Model file for the job. Use its own axes, mm. Face numbers are marked on the shaded views. A direction names the side the tool comes from. Give positions to 0.01 mm unless a question says otherwise; leave off trailing zeros. Write each loop counter-clockwise with the first axis right and the second up, starting at its lowest first coordinate (ties: lowest second). Pieces come first, ordered by that corner, then holes.
Autodesk Inventor part; units mm, degrees
ref_plane "YZ Plane" through (0, 0, 0) normal (1, 0, 0) x (0, 1, 0)
ref_plane "XZ Plane" through (0, 0, 0) normal (0, 1, 0) x (-1, 0, 0)
ref_plane "XY Plane" through (0, 0, 0) normal (0, 0, 1) x (1, 0, 0)
sketch "Sketch1" plane through (0, 0, 0) normal (0, 0, 1) x (1, 0, 0)
  line L0 (-292.1, -444.5) -> (292.1, -444.5)
  line L1 (292.1, -444.5) -> (292.1, 444.5)
  line L2 (292.1, 444.5) -> (-292.1, 444.5)
  line L3 (-292.1, 444.5) -> (-292.1, -444.5)
  line L4 (-292.1, -444.5) -> (292.1, 444.5) construction
  line L5 (292.1, -444.5) -> (-292.1, 444.5) construction
  line L6 (-309.626, 462.026) -> (309.626, 462.026)
  line L7 (309.626, 462.026) -> (309.626, -462.026)
  line L8 (309.626, -462.026) -> (-309.626, -462.026)
  line L9 (-309.626, -462.026) -> (-309.626, 462.026)
  point P0 (0, 0)
  dimension "d0" = 584.2
  dimension "d1" = 889
  dimension "d4" = 17.526
extrude "Extrusion1" add sketch "Sketch1" against normal blind 438.15 contours L3 L2 L1 L0 | L6 L7 L8 L9
extrude "Extrusion2" cut sketch "Sketch1" against normal blind 431.8 contours L3 L2 L1 L0
sketch "Sketch3" plane through (-309.626, -462.026, 0) normal (-1, 0, 0) x (0, 0, 1)
  line L0 (0, 0) -> (-438.15, 0) construction
  line L1 (-438.15, 0) -> (-438.15, 924.052) construction
  line L2 (-438.15, 924.052) -> (0, 924.052) construction
  line L3 (0, 924.052) -> (0, 0) construction
  line L4 (-38.1, 600.456) -> (-151.13, 600.456) construction
  line L5 (-56.896, 619.252) -> (-132.334, 619.252)
  line L6 (-132.334, 581.66) -> (-56.896, 581.66)
  arc A0 (-56.896, 581.66) -> (-56.896, 619.252) centre (-56.896, 600.456) ccw
  arc A1 (-132.334, 619.252) -> (-132.334, 581.66) centre (-132.334, 600.456) ccw
  line L7 (-287.02, 600.456) -> (-400.05, 600.456) construction
  line L8 (-305.816, 619.252) -> (-381.254, 619.252)
  line L9 (-381.254, 581.66) -> (-305.816, 581.66)
  arc A2 (-305.816, 581.66) -> (-305.816, 619.252) centre (-305.816, 600.456) ccw
  arc A3 (-381.254, 619.252) -> (-381.254, 581.66) centre (-381.254, 600.456) ccw
  point P0 (0, 462.026)
  point P1 (-94.615, 600.456)
  point P2 (-343.535, 600.456)
  point P3 (-38.1, 600.456)
  point P4 (-400.05, 600.456)
  dimension "d7" = 113.03
  dimension "d8" = 37.592
  dimension "d9" = 113.03
  dimension "d10" = 38.1
  dimension "d11" = 304.8
  dimension "d12" = 38.1
extrude "Extrusion3" cut sketch "Sketch3" against normal through all
equation "\"d9\" = d7"
properties part number "old battery cart" material "Wood (Birch)"
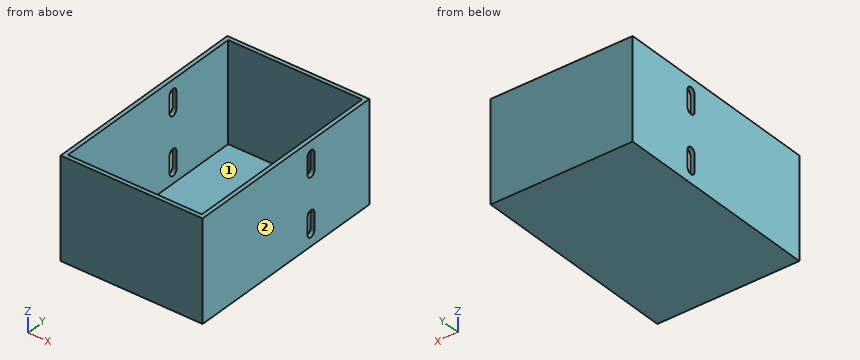
1. Probe probe 1 along X at (y, z) = (-327, -124); probe 2 along Y at (x, z) = (-73.5, -61); probe 3 along Z at (x, y) = (-145.5, -216). List the from-to ranges inside material, lowest first.
Calculated:
probe 1: x = -309.63 to -292.1, 292.1 to 309.63
probe 2: y = -462.03 to -444.5, 444.5 to 462.03
probe 3: z = -438.15 to -431.8
2. Pin check, flat tip, straight feed: P1, Ø3, axis at x = -23.5, y = 138.5, coming from the +Z side. Stop position of the tip, or through.
Calculated:
P1: stops at z = -431.8
3. Slice it at A-A, the plane y = 138.43. Write the cut outline in (x, z).
Calculated:
outline: (-309.63, -438.15) - (309.63, -438.15) - (309.63, -400.05) - (292.1, -400.05) - (292.1, -431.8) - (-292.1, -431.8) - (-292.1, -400.05) - (-309.63, -400.05) - close; (-309.63, -287.02) - (-292.1, -287.02) - (-292.1, -151.13) - (-309.63, -151.13) - close; (-309.63, -38.1) - (-292.1, -38.1) - (-292.1, 0) - (-309.63, 0) - close; (292.1, -287.02) - (309.63, -287.02) - (309.63, -151.13) - (292.1, -151.13) - close; (292.1, -38.1) - (309.63, -38.1) - (309.63, 0) - (292.1, 0) - close
4. Which spindle directions (+Z, -Z, +X, -X, +Y, -Y) get a long thin tool onto all of the face, cutting with end or side? Do the marked faces 1 and 2. Say none if no direction does.
Calculated:
face 1: +Z
face 2: +Z, -Z, +X, +Y, -Y
5. Slice it at B-B, the plane z = -165.5. Write the cut outline in (x, y).
Calculated:
outline: (-309.63, -462.03) - (309.63, -462.03) - (309.63, 462.03) - (-309.63, 462.03) - close; hole (-292.1, -444.5) - (292.1, -444.5) - (292.1, 444.5) - (-292.1, 444.5) - close
6. Slice it at C-C, the plane x = 54. Write the cut outline in (y, z).
Calculated:
outline: (-462.03, -438.15) - (462.03, -438.15) - (462.03, 0) - (444.5, 0) - (444.5, -431.8) - (-444.5, -431.8) - (-444.5, 0) - (-462.03, 0) - close
